```python
from build123d import *

# Parameters (mm, degrees)
FRONT_PLANE_EXTRUDED_BOSS_DEPTH       = 83
SMALLER_TRIANGULAR_EXTRUDED_CUT_DEPTH = 122.136286884
BIGGER_TRIANGULAR_EXTRUDED_CUT_DEPTH  = 122.136286884
F_19_075D_HOLE_D                      = 19.07499995
DOVETAIL_EXTRUDED_CUT_DEPTH           = 106.52963508
DOVETAIL_EXTRUDED_CUT_DEPTH_BACK      = 106.52963508


with BuildPart() as part:
    # Sketch4 → Front Plane Extruded Boss (new body)
    with BuildSketch(Plane.XY):
        Polygon((14.6, 0), (-14, 0), (-14, 6), (-27, 6), (-27, 84), (27, 84), (27, 6), (14.6, 6), align=None)
    extrude(amount=FRONT_PLANE_EXTRUDED_BOSS_DEPTH)

    # Sketch5 → Smaller Triangular Extruded Cut (cut, through all)
    with BuildSketch(Plane.XY.offset(83)):
        Polygon((-27, 84), (-8, 84), (-27, 68.057107008), align=None)
    extrude(amount=-SMALLER_TRIANGULAR_EXTRUDED_CUT_DEPTH, mode=Mode.SUBTRACT)

    # Sketch6 → Bigger Triangular Extruded Cut (cut, through all)
    with BuildSketch(Plane.XY.offset(83)):
        Polygon((27, 84), (-8, 84), (27, 42.288624259), align=None)
    extrude(amount=-BIGGER_TRIANGULAR_EXTRUDED_CUT_DEPTH, mode=Mode.SUBTRACT)

    # 19.075D Hole (through all)
    with Locations(Plane(origin=(27, 0, 0), x_dir=(0, 0, -1), z_dir=(1, 0, 0))):
        with Locations((-61, 22)):
            Hole(F_19_075D_HOLE_D / 2)

    # Sketch13 → Dovetail Extruded Cut (cut, two sides: drawn at the far end of the back side and taken through both)
    with BuildSketch(Plane(origin=(-8, 84, 53.436914958), x_dir=(0.8307334510088613, 0.4445504234012626, 0.3350475405500927), z_dir=(-0.5566703992264255, 0.6634139481689373, 0.49999999999999484)).offset(-DOVETAIL_EXTRUDED_CUT_DEPTH_BACK)):
        Polygon((0, 0), (-12.600448024, 1.600638285), (-2.270103373, -23.021812416), (5.416314056, -12.909823471), align=None)
    extrude(amount=DOVETAIL_EXTRUDED_CUT_DEPTH + DOVETAIL_EXTRUDED_CUT_DEPTH_BACK, mode=Mode.SUBTRACT)


solid = part.part
```
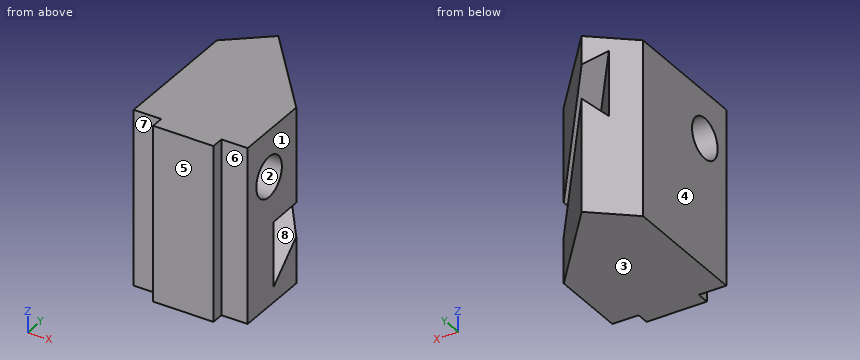
Check sheet for the modelled part. Datum: model origin and axes. Units: mm. Face numbers are marked on the shaded views. A direction names the side the tool comes from. Round coordinates to 2 decimals unless told otherwise and drop trailing zeros. Loops run counter-clockwise (first coordinate to the right, second up) from the corner with the lowest first, then second, coordinate; pieces in that order, holes last. Notation, with made-up numbers: (-13, 66) -> (16, 66) arc R11 cw to (16, 82) -> close; hole circle Ø1 at (18, 35.5). An arc over 180 degrees is marked (long way). Write item = value, one per line. Start each with the question number.
1) Sectioned sample at C-C, the plane x = -10.5. Record the cut outline in (y, z) (1 decimal).
2) Set-up check for the marked faces 4, 5, 6, 7 and 8: record each of +Z, -Z, +X, -X, +Y, -Y from which the full face is reachable in a straight line by a thin tool's end or side.
3) Thickness scan on probe 1 along Z at (x, y) = (3.5, 59.5); probe 2 along Y at (x, z) = (15, 57.5); probe 3 along Z at (x, y) = (3, 58). Record the ranges inside material, lowest first.
4) Sectioned sample at A-A, the plane y = 22. Record the cut outline in (x, z).
5) Sectioned sample at D-D, the plane z = 61. Record the cut outline in (x, y), plus the area to 3 significant figures.
6) Gauge pin test, flat ends, axial feed: pin 1 Ø1 at (x, z) = (20.5, 17) entering from +Y; pin 2 Ø2 at (x, z) = (-21, 50) entering from +Y; pin 3 Ø3 at (y, z) = (2.5, 49.5) entering from -X. Record the tip position at first contact, or that the pin passes through.
7) Release check for a two-part mould opening along Z. For the marked faces 1, 2 and 3 record: released by +Z, released by -Z, zero draft, split by the parting line, or undercut.
8) Sectioned sample at B-B, the plane z = 49.5. Record the cut outline in (x, y), plus the area to 3 significant figures.
Results are:
q1.outline = (0, 0) -> (81.9, 0) -> (81.9, 51.3) -> (69.9, 40.8) -> (69.9, 71.6) -> (81.9, 71.8) -> (81.9, 83) -> (0, 83) -> close; hole circle Ø19.1 at (22, 61)
q2.face_4 = +Z, -Z, -X, +Y, -Y
q2.face_5 = +Z, -Z, +X, -X, -Y
q2.face_6 = +Z, -Z, +X, -Y
q2.face_7 = +Z, -Z, -X, -Y
q2.face_8 = none
q3.probe_1 = 0 to 33.71, 59.13 to 83
q3.probe_2 = 6 to 13.13, 30.87 to 56.59
q3.probe_3 = 0 to 32.33, 59.55 to 83
q4.outline = (-27, 0) -> (27, 0) -> (27, 51.46) -> (-27, 51.46) -> close; (-27, 70.54) -> (27, 70.54) -> (27, 83) -> (-27, 83) -> close
q5.outline = (-27, 6) -> (-14, 6) -> (-14, 0) -> (14.6, 0) -> (14.6, 6) -> (27, 6) -> (27, 12.46) -> (-27, 12.46) -> close; (-27, 31.54) -> (27, 31.54) -> (27, 42.29) -> (1.58, 72.59) -> (1.32, 55.78) -> (-16.43, 76.93) -> (-27, 68.06) -> close
q5.area = 2,240 mm^2
q6.pin_1 = 50.63
q6.pin_2 = 73.93
q6.pin_3 = -14
q7.face_1 = zero draft
q7.face_2 = undercut
q7.face_3 = released by -Z
q8.outline = (-27, 6) -> (-14, 6) -> (-14, 0) -> (14.6, 0) -> (14.6, 6) -> (27, 6) -> (27, 42.29) -> (14.38, 57.33) -> (14.12, 40.53) -> (-16.43, 76.93) -> (-27, 68.06) -> close; (-12.52, 80.2) -> (-3.62, 78.78) -> (-8, 84) -> close
q8.area = 3,070 mm^2
